Verification items for the finished model (mm, model axes). Round coordinates to 2 decimals unless told otherwise and drop trailing zeros. Use a Markdown table: item, result. Add a question column.
Autodesk Inventor part; units mm, degrees
ref_plane "XZ Plane" through (0, 0, 0) normal (0, 1, 0) x (-1, 0, 0)
ref_plane "XY Plane" through (0, 0, 0) normal (0, 0, 1) x (1, 0, 0)
sketch "Sketch1" plane through (0, 0, 0) normal (0, 1, 0) x (-1, 0, 0)
  line L0 (-15, 15) -> (15, 15)
  line L1 (15, 15) -> (15, -15)
  line L2 (15, -15) -> (-15, -15)
  line L3 (-15, -15) -> (-15, 15)
  line L4 (-15, 15) -> (15, -15) construction
  line L5 (15, 15) -> (-15, -15) construction
  point P0 (0, 0)
  dimension "d0" = 30
  dimension "d1" = 30
extrude "Extrusion1" add sketch "Sketch1" along normal blind 14
sketch "Sketch2" plane through (0, 14, 0) normal (0, 1, 0) x (1, 0, 0)
  point P0 (0, 0)
  point P1 (0, 0)
sketch "Sketch3" plane through (0, 0, 0) normal (1, 0, 0) x (0, 1, 0)
  line L0 (14, -15) -> (14, 15) construction
  line L1 (14, 0) -> (14, -6.5) construction
  line L2 (14, 0) -> (14, -6.5)
  line L3 (14, 0) -> (10, 0) construction
  line L4 (14, 0) -> (11, 0) construction
  line L5 (11, 0) -> (11, -4) construction
  line L6 (11, 0) -> (12.25, 0) construction
  line L7 (12.25, 0) -> (12.25, -5.5) construction
  line L8 (10, 0) -> (10, 1) construction
  line L9 (14, 0) -> (13.5, 0) construction
  line L10 (13.5, 0) -> (13.5, -6.25) construction
  arc A0 (10, 0) -> (11, -4) centre (18.5, 0) ccw
  arc A1 (11, -4) -> (12.25, -5.5) centre (15.2361, -1.7407) ccw
  arc A2 (12.25, -5.5) -> (13.5, -6.25) centre (15.7243, -1.1261) ccw
  line L11 (13.5, -6.25) -> (14, -6.5)
  line L12 (14, 0) -> (10, 0)
  line L13 (-3.7, 0) -> (22.2, 0)
  point P0 (0, 0)
  dimension "d4" = 6.5
  dimension "d5" = 4
  dimension "d6" = 3
  dimension "d7" = 4
  dimension "d8" = 1.25
  dimension "d9" = 5.5
  dimension "d10" = 1
  dimension "d11" = 0.5
  dimension "d12" = 6.25
revolve "Revolution1" cut sketch "Sketch3" angle 360 about axis through (0, -10, 0) along (0, 1, 0)
sketch "Sketch4" plane through (0, 14, 0) normal (0, 1, 0) x (1, 0, 0)
  line L0 (0, 0) -> (0, 2) construction
  line L1 (0, 2) -> (0, -2) construction
  dimension "d14" = 2
  dimension "d15" = 4
hole "Hole1" at (0, 14, 2) at (0, 14, -2) direction (0, -1, 0) diameter 1.5 depth 100 tip angle 118
properties part number "ProxFinger_Mold"
1. Scan lines: line 1 along Z through (x, y) = (0, 3.75); line 2 along X through (y, z) = (8, 2); line 3 along Z through (x, y) = (5.25, 12.75). Record each from-to range of solid material in increasing order. Write a range as from..to.
2. Cross-section at A-A on x = 0. Count the separate pieces of the cut face and the enclosed holes in it, plus the area to 3 significant figures.
3. Release check for a two-part mould opening along Z. For faces 1 (the cylindrical face through (0.29, 5.16, 2.69)), 2 (the flat face through (-15, 7, 0)), 3 (the flat face through (0, 7, -15)), 4 (the cylindrical face through (0.29, 5.16, -1.31)) record: +Z half, -Z half, draft (parallel to the pull), parting line (faces both ways), or undercut.
4. Depth check by flat-ended pin: pin 1 Ø1.7 at (x, z) = (0, -2) entering from +Y. Enter the tip coordinate at first touch or a pass-through.
Answer:
| question | item | result |
|---|---|---|
| 1 | line 1 | z = -15..-2.75, -1.25..1.25, 2.75..15 |
| 1 | line 2 | x = -15..-0.75, 0.75..15 |
| 1 | line 3 | z = -15..-2.59, 2.59..15 |
| 2 | separate pieces | 3 |
| 2 | enclosed holes | 0 |
| 2 | area | 351 mm^2 |
| 3 | face 1 | undercut |
| 3 | face 2 | draft |
| 3 | face 3 | -Z half |
| 3 | face 4 | undercut |
| 4 | pin 1 | stops at y = 10.49 |
